from build123d import *

# Parameters (mm, degrees)
F0_R            = 45
F1_DEPTH        = 3
F2_R            = 3.25
F3_DEPTH        = 25
F3_COPIES_COUNT = 6


# Not quite as in the source:
# - a pattern or mirror of a feature is missing from the dataset's text; its kind, count and spacing are read off the source's solid


with BuildPart() as f1:
    # F0 (on Front) → F1 (new body, symmetric)
    with BuildSketch(Plane.XZ):
        Circle(F0_R)
    extrude(amount=F1_DEPTH, both=True)

    # F2 (on face) → F3 (cut)
    with BuildSketch(Plane.XZ.offset(3)):
        with Locations((0, 37)):
            Circle(F2_R)
    f3 = extrude(amount=-F3_DEPTH, mode=Mode.SUBTRACT)

    # F3_copies: F3 ×6 about axis
    f3_copies_axis = Axis((0, 0, 0), (0, 1, 0))
    for i in range(1, F3_COPIES_COUNT):
        add(f3.rotate(f3_copies_axis, i * 360 / F3_COPIES_COUNT), mode=Mode.SUBTRACT)


solid = f1.part
Design review of the part built by this model. Coordinates are the model's own, in mm. Round coordinates to 2 decimals unless told otherwise and drop trailing zeros. Write each loop counter-clockwise with the first axis right and the second up, starting at its lowest first coordinate (ties: lowest second). Pieces come first, ordered by that corner, then holes. Notation, with made-up numbers: (-6, 69.25) - (16, 69.25) arc R20 ccw to (16, 93.25) - close; hole circle Ø3 at (43.5, 13.25). An arc over 180 degrees is marked (long way). Return JSON: item names as keys, results as strings. Group by question number.
Item 1: We need section D-D on z = -37. Write out the cut boundary in (x, y).
Item 2: The part is to be moulded in two halves that separate along Z. For faces 1 (the face through (30.296, -0.042, 15.76)), 2 (the face through (-1, -3, 1)), 3 (the face through (20.765, -0.042, -39.923)), say which applies: pulls with the +Z half, pulls with the -Z half, needs draft (parallel to the pull), parting line crosses it, or undercut.
Item 3: Insertion check: P1, Ø3, axis at y = 2, z = -4, coming from the +X side; P2, Ø1, axis at y = -1, z = -7.5, coming from the -X side; P3, Ø1.5, axis at x = 19.5, y = -1, coming from the -Z side. Each pin has a flat end and moves straight along its axis. Give the tip position at first contact, or say it passes through.
Item 4: For probe 1 along Z at (x, y) = (0, 1.3); probe 2 along Z at (x, y) = (-33.5, 2.05); probe 3 along X at (y, z) = (1.75, 18), list the stretches that pass through material, from the lowest coordinate up. Write a range as [from, to].
Item 5: We need section C-C on y = 0.7. Write out the cut boundary in (x, z), and give its area (3 significant figures).
Item 6: We need section A-A on x = 0. Write out the cut boundary in (y, z), and give its area (3 significant figures).
Item 7: We need section B-B on z = -18.5. Write out the cut boundary in (x, y).
Model answer:
{
 "1": {"outline": "(-25.61, -3) - (-3.25, -3) - (-3.25, 3) - (-25.61, 3) - close; (3.25, -3) - (25.61, -3) - (25.61, 3) - (3.25, 3) - close"},
 "2": {"face 1": "undercut", "face 2": "needs draft", "face 3": "parting line crosses it"},
 "3": {"P1": "stops at x = 44.93", "P2": "stops at x = -44.45", "P3": "stops at z = -40.91"},
 "4": {"probe 1": "z = [-45, -40.25], [-33.75, 33.75], [40.25, 45]", "probe 2": "z = [-30.05, -21.41], [-15.59, 15.59], [21.41, 30.05]", "probe 3": "x = [-41.24, -35.25], [-28.83, 28.83], [35.25, 41.24]"},
 "5": {"outline": "circle Ø90 at (0, 0); hole circle Ø6.5 at (-32.04, -18.5); hole circle Ø6.5 at (-32.04, 18.5); hole circle Ø6.5 at (0, -37); hole circle Ø6.5 at (0, 37); hole circle Ø6.5 at (32.04, -18.5); hole circle Ø6.5 at (32.04, 18.5)", "area": "6,160 mm²"},
 "6": {"outline": "(-3, -45) - (3, -45) - (3, -40.25) - (-3, -40.25) - close; (-3, -33.75) - (3, -33.75) - (3, 33.75) - (-3, 33.75) - close; (-3, 40.25) - (3, 40.25) - (3, 45) - (-3, 45) - close", "area": "462 mm²"},
 "7": {"outline": "(-41.02, -3) - (-35.29, -3) - (-35.29, 3) - (-41.02, 3) - close; (-28.79, -3) - (28.79, -3) - (28.79, 3) - (-28.79, 3) - close; (35.29, -3) - (41.02, -3) - (41.02, 3) - (35.29, 3) - close"}
}
